from build123d import *

# Parameters (mm, degrees)
SALIENTE_EXTRUIR1_START             = -7.320816359
SALIENTE_EXTRUIR1_3_DEPTH           = 14.641632718
CROQUIS2_R                          = 8.293601056
SALIENTE_EXTRUIR2_DEPTH             = 0.996962704
CROQUIS3_R                          = 8.094208515
SALIENTE_EXTRUIR3_DEPTH             = 0.199392541
CROQUIS4_R                          = 8.293601056
SALIENTE_EXTRUIR4_DEPTH             = 2.099264862
CROQUIS6_R                          = 7.996393307
SALIENTE_EXTRUIR6_DEPTH             = 0.147505067
SALIENTE_EXTRUIR6_TAPER             = 67.466749921
CROQUIS7_R                          = 7.640868273
SALIENTE_EXTRUIR7_DEPTH             = 0.849457636
SALIENTE_EXTRUIR7_TAPER             = 22.533250079
DI_METRO_DE_TALADRO_12_0_12_1_D     = 12
DI_METRO_DE_TALADRO_12_0_12_1_DEPTH = 3
CHAFL_N1_SIZE                       = 0.598177622
CHAFL_N1_SIZE2                      = 0.601939746
CHAFL_N2_SIZE                       = 0.158849839
CHAFL_N2_SIZE_2                     = 0.292765242
REDONDEO1_R                         = 0.199050823


with BuildPart() as part:
    # Saliente-Extruir1: read off the stored shape, not the designer's step
    # Saliente-Extruir1 outline → Saliente-Extruir1 (revolve)
    with BuildSketch(Plane.YX):
        Polygon((8.99335601, -27.061359261), (0, -27.061359261), (0, -55.101016987), (8.244693452, -55.101016987), (8.244693452, -54.104054283), (7.443361166, -54.104054283), (7.443361166, -53.803084411), (8.244693452, -53.803084411), (8.244693452, -47.810021819), (8.99335601, -47.061359261), align=None)
    revolve(axis=Axis((0, 0, 0), (1, 0, 0)))

    # Saliente-Extruir1 2 outline → Saliente-Extruir1 2 (revolve)
    with BuildSketch(Plane.YX):
        Polygon((0, -55.101016987), (0, -63.6), (7.320816359, -63.6), (8.007236046, -59.33292836), (8.233407082, -55.101016987), align=None)
    revolve(axis=Axis((0, 0, 0), (1, 0, 0)))

    # Saliente-Extruir1 3 outline → Saliente-Extruir1 3 (cut)
    with BuildSketch(Plane.XY.offset(SALIENTE_EXTRUIR1_START)):
        Polygon((-63.6, 5.495125364), (-59.227359982, 6.566499061), (-55.157899775, 8.230367028), (-54, 8.70379403), (-54, 10), (-63.6, 10), align=None)
    extrude(amount=SALIENTE_EXTRUIR1_3_DEPTH, mode=Mode.SUBTRACT)

    # Croquis2 → Saliente-Extruir2 (add)
    with BuildSketch(Plane(origin=(-27.061359261, 0, 0), x_dir=(0, 0, -1), z_dir=(1, 0, 0))):
        Circle(CROQUIS2_R)
    extrude(amount=SALIENTE_EXTRUIR2_DEPTH)

    # Croquis3 → Saliente-Extruir3 (add)
    with BuildSketch(Plane(origin=(-26.064396557, 0, 0), x_dir=(0, 0, -1), z_dir=(1, 0, 0))):
        Circle(CROQUIS3_R)
    extrude(amount=SALIENTE_EXTRUIR3_DEPTH)

    # Croquis4 → Saliente-Extruir4 (add)
    with BuildSketch(Plane(origin=(-25.865004017, 0, 0), x_dir=(0, -1, 0), z_dir=(-1, 0, 0))):
        with Locations(Location((0, 0, 0), (0, 0, 270))):
            Circle(CROQUIS4_R)
    extrude(amount=-SALIENTE_EXTRUIR4_DEPTH)

    # Croquis6 → Saliente-Extruir6 (add)
    with BuildSketch(Plane(origin=(-23.765739154, 0, 0), x_dir=(0, 0, -1), z_dir=(1, 0, 0))):
        Circle(CROQUIS6_R)
    extrude(amount=SALIENTE_EXTRUIR6_DEPTH, taper=SALIENTE_EXTRUIR6_TAPER)

    # Croquis7 → Saliente-Extruir7 (add)
    with BuildSketch(Plane(origin=(-23.618234087, 0, 0), x_dir=(0, 0, -1), z_dir=(1, 0, 0))):
        Circle(CROQUIS7_R)
    extrude(amount=SALIENTE_EXTRUIR7_DEPTH, taper=SALIENTE_EXTRUIR7_TAPER)

    # Diámetro de taladro Ø12.0 (12)1
    with Locations(Plane(origin=(-22.768776451, 0, 0), x_dir=(0, 0, -1), z_dir=(1, 0, 0))):
        with Locations((0, 0)):
            Hole(DI_METRO_DE_TALADRO_12_0_12_1_D / 2, depth=DI_METRO_DE_TALADRO_12_0_12_1_DEPTH)

    # Chaflán1
    chafl_n1_edges = [part.edges().sort_by_distance(p)[0] for p in [
        (-27.061359261, -8.99335601, 0),
    ]]
    chafl_n1_side = [part.faces().sort_by_distance(p)[0] for p in [
        (-27.061359261, -8.738985489, 0),
    ]]
    chamfer(chafl_n1_edges, length=CHAFL_N1_SIZE, length2=CHAFL_N1_SIZE2, reference=chafl_n1_side[0])

    # Chaflán2
    # the kernel refuses this chamfer: 0.292765242, 0.158849839 mm, written as the material it takes off along each edge
    with BuildSketch(Plane(origin=(-22.768776451, 0, 0), x_dir=(0, 0, -1), z_dir=(0, 1, 0))) as chafl_n2_piece_1:
        Polygon((7.288433722 + CHAFL_N2_SIZE * 0.38321951697, CHAFL_N2_SIZE * 0.923657297312), (7.288433722 - CHAFL_N2_SIZE_2, 0), (7.288433722, 0), align=None)
    revolve(axis=Axis((-22.768776451, 0, 0), (-1, 0, 0)), mode=Mode.SUBTRACT)

    # Redondeo1
    redondeo1_edges = [part.edges().sort_by_distance(p)[0] for p in [
        (-23.765739154, 0, 8.293601056),
    ]]
    fillet(redondeo1_edges, radius=REDONDEO1_R)


solid = part.part
The listing builds one solid part. Answer for the finished solid, in the listing's coordinates (mm). A direction names the side the tool comes from. Give positions to 0.01 mm unless a question says otherwise; leave off trailing zeros. Write each loop counter-clockwise with the first axis right and the second up, starting at its lowest first coordinate (ties: lowest second). Pieces come first, ordered by that corner, then holes. Notation, with made-up numbers: (31, 43) -> (44, 43) arc R27 ccw to (44, 74) -> close; hole circle Ø7 at (24, 80.25). An arc over 180 degrees is marked (long way). Use a Markdown table: item, result.
(1) Flat-ended cylindrical pins translate along their axes: P1, Ø1, axis at x = -41, z = -4, coming from the +Y side; P2, Ø1, axis at x = -38.5, z = 6, coming from the -Y side; P3, Ø1, axis at x = -44, y = 2.5, coming from the -Z side. Find the tip coordinate at first contact, or state that the pin passes through.
Return value:
| item | result |
|---|---|
| P1 | y = 8.28 |
| P2 | y = -7.12 |
| P3 | z = -8.77 |
(2) Determine the mould class of faces 4 (the flat face through (-25.769, 0, 0)), 5 (the conical face through (-57.66, -8.09, 0.36)), 6 (the flat face through (-53.803, 1.9, 7.4)) for opening direction Z: released by +Z, released by -Z, zero draft, split by the parting line, or undercut.
Return value:
| item | result |
|---|---|
| face 4 | undercut |
| face 5 | split by the parting line |
| face 6 | zero draft |
(3) Section A-A, the plane x = -40 is taken. Determine the outline of the cut face in (y, z), then the cut area to 3 significant figures.
Return value:
| item | result |
|---|---|
| outline | circle Ø17.99 at (0, 0) |
| area | 254 mm2 |
(4) For faces 1 (the cylindrical face through (-50.765, -1.073, 8.175)), 2 (the cylindrical face through (-24.928, -0.365, 8.286)), 3 (the flat face through (-63.6, -1, 0)), determine the directions among +Z, -Z, +X, -X, +Y, -Y from which every point of the face is accessible in a straight line to the end or side of a thin tool.
Return value:
| item | result |
|---|---|
| face 1 | -X |
| face 2 | +X |
| face 3 | +Z, -Z, -X, +Y, -Y |
(5) Find the intervals of material crossed by probe 1 along Y at (x, z) = (-24.75, 0); probe 2 along X at (y, z) = (-2.25, 4); probe 3 along Y at (x, z) = (-35, 0.25), in increasing order. Write a range as from..to.
Return value:
| item | result |
|---|---|
| probe 1 | -8.29..-6, 6..8.29 |
| probe 2 | -63.6..-25.77 |
| probe 3 | -8.99..8.99 |
